Input: part model. Units: mm. Frame: model coordinates. Face numbers are marked on the shaded views. A direction names the side the tool comes from. Round coordinates to 2 decimals unless told otherwise and drop trailing zeros. Loops run counter-clockwise (first coordinate to the right, second up) from the corner with the lowest first, then second, coordinate; pieces in that order, holes last. Notation, with made-up numbers: (81, -9.75) - (112, -9.75) arc R19 cw to (112, 13.25) - close; hole circle Ø11 at (-12, -26.75). An arc over 180 degrees is marked (long way). Use CSV: the item, a comma, the result in double quotes. Start each with the question number.
1. Cut plane A-A (z = 20). Return loops of the section in (x, y).
2. Material intervals for probe 1 along X at (y, z) = (8.75, 35); probe 2 along X at (y, z) = (11.15, 40); probe 3 along Y at (x, z) = (-2.25, 36), sorted ascending. Write a range as from..to.
3. Cut plane D-D (y = 5.75). Return loops of the section in (x, z), and give its area (3 significant figures).
4. Access query for the marked faces 1 and 2. Directions: +Z, -Z, +X, -X, +Y, -Y. A direction counts if a zero-diameter tool reaches every point of the face in a straight line with its end or side. Return the directions, or none.
5. Cut plane B-B (x = 0). Return loops of the section in (y, z).
6. Cut plane C-C (z = 5.5). Return loops of the section in (x, y), and give its area (3 significant figures).
7. Pin query (flat end, axial travel): P1, Ø4, axis at x = 4.5, y = -1, coming from the +Z side; P2, Ø10, axis at x = -1, z = 13, coming from the -Y side. Return the tip coordinate at first contact, or that it passes through.
```python
from build123d import *

# Parameters (mm, degrees)
SKETCH2_W           = 26.4
SKETCH2_H           = 26.4
SKETCH2_W_2         = 20.4
SKETCH2_H_2         = 20.4
BOSS_EXTRUDE1_DEPTH = 50
SKETCH3_W           = 26.4
SKETCH3_H           = 26.4
BOSS_EXTRUDE2_DEPTH = 3
SKETCH4_W           = 20.4
SKETCH4_H           = 50
CUT_EXTRUDE1_DEPTH  = 3
SKETCH5_W           = 26.4
SKETCH5_H           = 53
CUT_EXTRUDE2_DEPTH  = 10
SKETCH6_R           = 1.25
CUT_EXTRUDE3_DEPTH  = 10


with BuildPart() as part:
    # Sketch2 → Boss-Extrude1 (new body)
    with BuildSketch(Plane.XY):
        Rectangle(SKETCH2_W, SKETCH2_H)
        Rectangle(SKETCH2_W_2, SKETCH2_H_2, mode=Mode.SUBTRACT)
    extrude(amount=BOSS_EXTRUDE1_DEPTH)

    # Sketch3 → Boss-Extrude2 (add)
    with BuildSketch(Plane(origin=(0, 0, 0), x_dir=(-1, 0, 0), z_dir=(0, 0, -1))):
        Rectangle(SKETCH3_W, SKETCH3_H)
    extrude(amount=BOSS_EXTRUDE2_DEPTH)

    # Sketch4 → Cut-Extrude1 (cut)
    with BuildSketch(Plane.XZ.offset(13.2)):
        with Locations((0, 25)):
            Rectangle(SKETCH4_W, SKETCH4_H)
    extrude(amount=-CUT_EXTRUDE1_DEPTH, mode=Mode.SUBTRACT)

    # Sketch5 → Cut-Extrude2 (cut)
    with BuildSketch(Plane.XZ.offset(13.2)):
        with Locations((0, 23.5)):
            Rectangle(SKETCH5_W, SKETCH5_H)
    extrude(amount=-CUT_EXTRUDE2_DEPTH, mode=Mode.SUBTRACT)

    # Sketch6 → Cut-Extrude3 (cut)
    with BuildSketch(Plane(origin=(0, 13.2, 0), x_dir=(1, 0, 0), z_dir=(0, 1, 0))):
        with Locations(Location((0, -20, 0), (0, 0, 270))):
            Circle(SKETCH6_R)
        with Locations(Location((0, -40, 0), (0, 0, 270))):
            Circle(SKETCH6_R)
    extrude(amount=-CUT_EXTRUDE3_DEPTH, mode=Mode.SUBTRACT)


solid = part.part
```
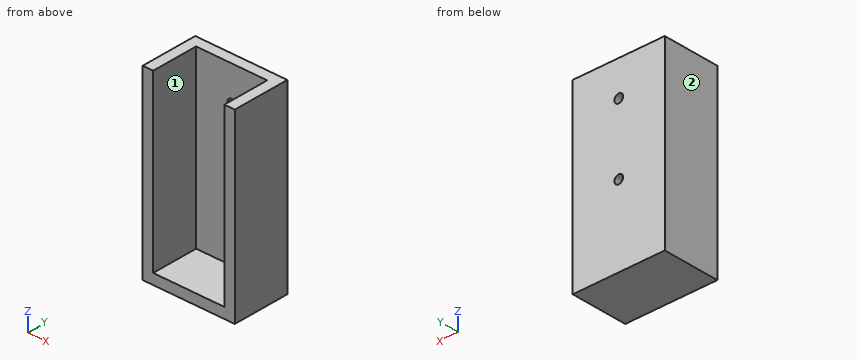
Established:
1,outline,"(-13.2, -3.2) - (-10.2, -3.2) - (-10.2, 10.2) - (-1.25, 10.2) - (-1.25, 13.2) - (-13.2, 13.2) - close; (1.25, 10.2) - (10.2, 10.2) - (10.2, -3.2) - (13.2, -3.2) - (13.2, 13.2) - (1.25, 13.2) - close"
2,probe 1,"x = -13.2..-10.2, 10.2..13.2"
2,probe 2,"x = -13.2..-1.25, 1.25..13.2"
2,probe 3,"y = 10.2..13.2"
3,outline,"(-13.2, -3) - (13.2, -3) - (13.2, 50) - (10.2, 50) - (10.2, 0) - (-10.2, 0) - (-10.2, 50) - (-13.2, 50) - close"
3,area,"379 mm2"
4,face 1,"+Z, -Y"
4,face 2,"+Z, -Z, -X, +Y, -Y"
5,outline,"(-3.2, -3) - (13.2, -3) - (13.2, 18.75) - (10.2, 18.75) - (10.2, 0) - (-3.2, 0) - close; (10.2, 21.25) - (13.2, 21.25) - (13.2, 38.75) - (10.2, 38.75) - close; (10.2, 41.25) - (13.2, 41.25) - (13.2, 50) - (10.2, 50) - close"
6,outline,"(-13.2, -3.2) - (-10.2, -3.2) - (-10.2, 10.2) - (10.2, 10.2) - (10.2, -3.2) - (13.2, -3.2) - (13.2, 13.2) - (-13.2, 13.2) - close"
6,area,"160 mm2"
7,P1,"stops at z = 0"
7,P2,"stops at y = 10.2"
